```python
from build123d import *

# Parameters (mm, degrees)
SKETCH_1_R      = 1.5
SKETCH_1_R_2    = 3.121318996
SKETCH_1_W      = 5.05
SKETCH_1_H      = 2.05
SKETCH_1_W_2    = 2.05
SKETCH_1_H_2    = 5.05
EXTRUDE_1_DEPTH = 2


with BuildPart() as part:
    # 草图1 → 凸台-拉伸1 (new body)
    with BuildSketch(Plane.XY):
        Polygon((-56.111334712, -13.372248853), (31.071025228, -13.372248853), (31.071025228, -137.372248853), (-56.111334712, -137.372248853), (-56.111334712, -152.372248853), (-56.111334712, -227.397248853), (62.919821756, -227.397248853), (62.919821756, -152.372248853), (62.919821756, 1.627751147), (-56.111334712, 1.627751147), align=None)
        with Locations((-19.586334712, -1.372248853)):
            Circle(SKETCH_1_R, mode=Mode.SUBTRACT)
        with Locations((20.413665288, -1.372248853)):
            Circle(SKETCH_1_R, mode=Mode.SUBTRACT)
        with Locations((-19.586334712, -149.372248853)):
            Circle(SKETCH_1_R, mode=Mode.SUBTRACT)
        with Locations((20.413665288, -149.372248853)):
            Circle(SKETCH_1_R, mode=Mode.SUBTRACT)
        with Locations((59.919821756, -97.372248853)):
            Circle(SKETCH_1_R, mode=Mode.SUBTRACT)
        with Locations((59.919821756, -57.372248853)):
            Circle(SKETCH_1_R, mode=Mode.SUBTRACT)
        with Locations((41.938665288, -93.678088908)):
            Circle(SKETCH_1_R_2, mode=Mode.SUBTRACT)
        with Locations((-19.586334712, -224.372248853)):
            Circle(SKETCH_1_R, mode=Mode.SUBTRACT)
        with Locations((20.413665288, -224.372248853)):
            Circle(SKETCH_1_R, mode=Mode.SUBTRACT)
        with Locations((39.413665288, -1.372248853)):
            Rectangle(SKETCH_1_W, SKETCH_1_H, mode=Mode.SUBTRACT)
        with Locations((49.413665288, -1.372248853)):
            Rectangle(SKETCH_1_W, SKETCH_1_H, mode=Mode.SUBTRACT)
        with Locations((-48.586334712, -1.372248853)):
            Rectangle(SKETCH_1_W, SKETCH_1_H, mode=Mode.SUBTRACT)
        with Locations((-38.586334712, -1.372248853)):
            Rectangle(SKETCH_1_W, SKETCH_1_H, mode=Mode.SUBTRACT)
        with Locations((39.413665288, -149.372248853)):
            Rectangle(SKETCH_1_W, SKETCH_1_H, mode=Mode.SUBTRACT)
        with Locations((49.413665288, -149.372248853)):
            Rectangle(SKETCH_1_W, SKETCH_1_H, mode=Mode.SUBTRACT)
        with Locations((-48.586334712, -149.372248853)):
            Rectangle(SKETCH_1_W, SKETCH_1_H, mode=Mode.SUBTRACT)
        with Locations((-38.586334712, -149.372248853)):
            Rectangle(SKETCH_1_W, SKETCH_1_H, mode=Mode.SUBTRACT)
        with Locations((59.919821756, -38.372248853)):
            Rectangle(SKETCH_1_W_2, SKETCH_1_H_2, mode=Mode.SUBTRACT)
        with Locations((59.919821756, -28.372248853)):
            Rectangle(SKETCH_1_W_2, SKETCH_1_H_2, mode=Mode.SUBTRACT)
        with Locations((59.919821756, -126.372248853)):
            Rectangle(SKETCH_1_W_2, SKETCH_1_H_2, mode=Mode.SUBTRACT)
        with Locations((59.919821756, -116.372248853)):
            Rectangle(SKETCH_1_W_2, SKETCH_1_H_2, mode=Mode.SUBTRACT)
        with Locations((39.413665288, -224.372248853)):
            Rectangle(SKETCH_1_W, SKETCH_1_H, mode=Mode.SUBTRACT)
        with Locations((49.413665288, -224.372248853)):
            Rectangle(SKETCH_1_W, SKETCH_1_H, mode=Mode.SUBTRACT)
        with Locations((-48.586334712, -224.372248853)):
            Rectangle(SKETCH_1_W, SKETCH_1_H, mode=Mode.SUBTRACT)
        with Locations((-38.586334712, -224.372248853)):
            Rectangle(SKETCH_1_W, SKETCH_1_H, mode=Mode.SUBTRACT)
    extrude(amount=EXTRUDE_1_DEPTH)


solid = part.part
```
Input: part model. Units: mm. Frame: model coordinates. Coordinates: 2 decimals unless noted, no trailing zeros. Loops run counter-clockwise (first coordinate to the right, second up) from the corner with the lowest first, then second, coordinate; pieces in that order, holes last.
Q1. Contact query for a flat-ended pin moving along its axis: pin 1 (0.6 mm diameter, centred on y = -28, z = 1, fed in from -X). Output: stop coordinate, or through.
Results are:
pin 1: stops at x = 31.07
Q2. Section A-A, the plane x = -32.5. Return the cut outline in (y, z), and give its area (3 significant figures).
Results are:
outline: (-227.4, 0) - (-137.37, 0) - (-137.37, 2) - (-227.4, 2) - close; (-13.37, 0) - (1.63, 0) - (1.63, 2) - (-13.37, 2) - close
area: 210 mm2
Q3. Line query: line 1 along Y through (x, z) = (9.5, 1.5); line 2 along Y through (x, z) = (-19, 1.8); line 3 along X through (y, z) = (-107.5, 1.45). Output: solid intervals per line, ascending.
Results are:
line 1: y = -227.4 to -137.37, -13.37 to 1.63
line 2: y = -227.4 to -225.75, -222.99 to -150.75, -147.99 to -137.37, -13.37 to -2.75, 0.01 to 1.63
line 3: x = 31.07 to 62.92
Q4. Section C-C, the plane z = 0.75. Give the number of separate pieces and of enclosed holes in the cut face, and give its area (3 significant figures).
Results are:
separate pieces: 1
enclosed holes: 25
area: 16,200 mm2
Q5. Section B-B, the plane y = -87. Return the cut outline in (x, z).
Results are:
outline: (31.07, 0) - (62.92, 0) - (62.92, 2) - (31.07, 2) - close
Q6. Mould query, pull axis Y, two halves, no side actions, for faces 1 (the flat face through (42, -137, 2)), 2 (the cylindrical face through (39.638, -91.569, 0.986)). Classes: +Y half, -Y half, draft (parallel to the pull), parting line (faces both ways), or undercut.
Results are:
face 1: draft
face 2: undercut
